from build123d import *

# Parameters (mm, degrees)
F0_W      = 304.8
F0_H      = 304.8
F1_DEPTH  = 304.8
F2_T      = -12.7
F3_W      = 279.4
F3_H      = 12.7
F4_DEPTH  = 292.1
F5_R      = 1.905
F6_DEPTH  = 12.7
F7_R      = 1.905
F8_DEPTH  = 41.275
F9_R      = 1.905
F10_DEPTH = 41.275
F11_R     = 1.905
F12_DEPTH = 41.275
F13_W     = 12.7
F13_H     = 83.6831671771
F14_DEPTH = 292.1
F15_R     = 1.905
F16_DEPTH = 41.275


with BuildPart() as f1:
    # F0 (on Front) → F1 (new body)
    with BuildSketch(Plane.XZ):
        with Locations((-0.2428255975, 39.7985728923)):
            Rectangle(F0_W, F0_H)
    extrude(amount=F1_DEPTH)

    # F2
    f2_openings = [f1.faces().sort_by_distance(p)[0] for p in [
        (-0.242826, 0, 39.798573),
    ]]
    offset(amount=F2_T, openings=f2_openings)

    # F3 (on face) → F4 (join)
    with BuildSketch(Plane(origin=(0, -292.1, 0), x_dir=(-1, 0, 0), z_dir=(0, 1, 0))):
        with Locations((0.2428255975, -9.8682599306)):
            Rectangle(F3_W, F3_H)
    extrude(amount=F4_DEPTH)

    # F5 (on face) → F6 (cut, symmetric)
    with BuildSketch(Plane.XY.offset(192.1985728923)):
        with Locations((-0.2428255975, -166.3160324097)):
            Circle(F5_R)
    extrude(amount=F6_DEPTH, both=True, mode=Mode.SUBTRACT)

    # F7 (on face) → F8 (cut)
    with BuildSketch(Plane.YZ.offset(152.1571744025)):
        with Locations((-254, -9.8682599306)):
            Circle(F7_R)
        with Locations((-177.8, -9.8682599306)):
            Circle(F7_R)
        with Locations((-101.6, -9.8682599306)):
            Circle(F7_R)
        with Locations((-25.4, -9.8682599306)):
            Circle(F7_R)
    extrude(amount=-F8_DEPTH, mode=Mode.SUBTRACT)

    # F9 (on face) → F10 (cut)
    with BuildSketch(Plane(origin=(-152.6428255975, 0, 0), x_dir=(0, -1, 0), z_dir=(-1, 0, 0))):
        with Locations((25.4, -9.6651343237)):
            Circle(F9_R)
        with Locations((101.6, -9.6651343237)):
            Circle(F9_R)
        with Locations((177.8, -9.6651343237)):
            Circle(F9_R)
        with Locations((254, -9.6629047766)):
            Circle(F9_R)
    extrude(amount=-F10_DEPTH, mode=Mode.SUBTRACT)

    # F11 (on face) → F12 (cut)
    with BuildSketch(Plane.XZ.offset(304.8)):
        with Locations((-89.1428255975, -9.7314271077)):
            Circle(F11_R)
        with Locations((-43.4228255975, -9.7314271077)):
            Circle(F11_R)
        with Locations((-0.2428255975, -9.7314271077)):
            Circle(F11_R)
        with Locations((42.9371744025, -9.7314271077)):
            Circle(F11_R)
        with Locations((88.6571744025, -9.7314271077)):
            Circle(F11_R)
    extrude(amount=-F12_DEPTH, mode=Mode.SUBTRACT)

    # F13 (on face) → F14 (join)
    with BuildSketch(Plane(origin=(0, -292.1, 0), x_dir=(-1, 0, 0), z_dir=(0, 1, 0))):
        with Locations((0.2428255975, -58.0598435192)):
            Rectangle(F13_W, F13_H)
    extrude(amount=F14_DEPTH)

    # F15 (on face) → F16 (cut)
    with BuildSketch(Plane.XY.offset(-3.5182599306)):
        with Locations((-0.2428255975, -31.75)):
            Circle(F15_R)
        with Locations((-0.2428255975, -146.05)):
            Circle(F15_R)
    extrude(amount=-F16_DEPTH, mode=Mode.SUBTRACT)


solid = f1.part
Geometry check sheet. Reference: the model listing, model coordinates, mm. A direction names the side the tool comes from. Round coordinates to 2 decimals unless told otherwise and drop trailing zeros. Order: outer loops, then holes, each group sorted by start corner. A loop starts at its lowest first (then second) coordinate and runs counter-clockwise, first axis right, second up. Notation, with made-up numbers: M 68.5,-16 L 124.5,-16 A35 ccw 124.5,22 Z; hole C 89.5,74 d6. An arc over 180 degrees is marked long. Write each question's results on one line, items separated by ' | '. Start each with the question number.
1. Go/stop test with flat-tipped pins: P1, Ø25, axis at x = 69.5, z = -58.5, coming from the +Y side; P2, Ø2.5, axis at y = -101.6, z = -9.67, coming from the -X side; P3, Ø2.5, axis at y = -25.4, z = -9.67, coming from the +X side. Record where each tip stops, or that it passes through.
2. Set-up check for faces 4 (the face through (-2, -150, -112.601)), 5 (the face through (6.107, -148, -59)): record each of +Z, -Z, +X, -X, +Y, -Y from which the full face is reachable in a straight line by a thin tool's end or side.
3. Cross-section at A-A on y = -215.5. Record the boundary of the cut face in (x, z), plus the area to 3 significant figures.
4. Cross-section at D-D on x = 128. Record the boundary of the cut face in (y, z) (3 decimals).
5. Material ranges on L1, parallel to X at y = -283, z = -94.5; L2, parallel to Z at x = -120, y = -101.6; L3, parallel to Z at x = 106, y = -51.5, recorded low to high. Write a range as from..to.
6. Cross-section at C-C on x = -80. Record the boundary of the cut face in (y, z).
7. Draft check along X on faces 1 (the face through (-152.643, -150, 38)), 2 (the face through (-2, -304.8, 42)), 3 (the face through (-2, -144, 179.499)). Enter one of: pulls with the +X half, pulls with the -X half, needs draft (parallel to the pull), parting line crosses it, or undercut.
8. Cross-section at B-B on z = -82.5. Record the boundary of the cut face in (x, y), plus the area to 3 significant figures.
Resolved:
1) P1: y = -292.1 | P2: x = -111.37 | P3: x = 110.88
2) face 4: -Z, +X, -X, +Y, -Y | face 5: +Y
3) outline: M -152.64,-112.6 L 152.16,-112.6 L 152.16,192.2 L -152.64,192.2 Z; hole M -139.94,-99.9 L -6.59,-99.9 L -6.59,-16.22 L -139.94,-16.22 Z; hole M -139.94,-3.52 L 139.46,-3.52 L 139.46,179.5 L -139.94,179.5 Z; hole M 6.11,-99.9 L 139.46,-99.9 L 139.46,-16.22 L 6.11,-16.22 Z | area: 19,400 mm2
4) outline: M -304.8,-112.601 L 0,-112.601 L 0,-99.901 L -292.1,-99.901 L -292.1,-16.218 L 0,-16.218 L 0,-3.518 L -292.1,-3.518 L -292.1,179.499 L 0,179.499 L 0,192.199 L -304.8,192.199 Z; hole C -254,-9.868 d3.81; hole C -177.8,-9.868 d3.81; hole C -101.6,-9.868 d3.81; hole C -25.4,-9.868 d3.81
5) L1: -152.64..-139.94, -6.59..6.11, 139.46..152.16 | L2: -112.6..-99.9, -16.22..-11.57, -7.76..-3.52, 179.5..192.2 | L3: -112.6..-99.9, -16.22..-3.52, 179.5..192.2
6) outline: M -304.8,-112.6 L 0,-112.6 L 0,-99.9 L -292.1,-99.9 L -292.1,-16.22 L 0,-16.22 L 0,-3.52 L -292.1,-3.52 L -292.1,179.5 L 0,179.5 L 0,192.2 L -304.8,192.2 Z
7) face 1: pulls with the -X half | face 2: needs draft | face 3: undercut
8) outline: M -152.64,-304.8 L 152.16,-304.8 L 152.16,0 L 139.46,0 L 139.46,-292.1 L 6.11,-292.1 L 6.11,0 L -6.59,0 L -6.59,-292.1 L -139.94,-292.1 L -139.94,0 L -152.64,0 Z | area: 15,000 mm2
